from build123d import *

# Parameters (mm, degrees)
F0_W     = 350
F0_H     = 1250
F0_W_2   = 60
F0_H_2   = 48
F0_W_3   = 60.0317394733
F0_W_4   = 27
F0_H_3   = 72
F1_DEPTH = 60


with BuildPart() as f1:
    # F0 (on Front) → F1 (new body)
    with BuildSketch(Plane.XZ):
        with Locations((-0.2704625484, 126.1477753774)):
            Rectangle(F0_W, F0_H)
        with Locations((-95, -116)):
            Rectangle(F0_W_2, F0_H_2, mode=Mode.SUBTRACT)
        with Locations((-95, -49)):
            Rectangle(F0_W_2, F0_H_2, mode=Mode.SUBTRACT)
        with Locations((-95.0158697367, 18)):
            Rectangle(F0_W_3, F0_H_2, mode=Mode.SUBTRACT)
        with Locations((95, -116)):
            Rectangle(F0_W_2, F0_H_2, mode=Mode.SUBTRACT)
        with Locations((95, -49)):
            Rectangle(F0_W_2, F0_H_2, mode=Mode.SUBTRACT)
        with Locations((95.0158697367, 18)):
            Rectangle(F0_W_3, F0_H_2, mode=Mode.SUBTRACT)
        with Locations((-95.0158697367, 85)):
            Rectangle(F0_W_3, F0_H_2, mode=Mode.SUBTRACT)
        with Locations((-95.0158697367, 152)):
            Rectangle(F0_W_3, F0_H_2, mode=Mode.SUBTRACT)
        with Locations((-95.0158697367, 219)):
            Rectangle(F0_W_3, F0_H_2, mode=Mode.SUBTRACT)
        with Locations((-95.0158697367, 286)):
            Rectangle(F0_W_3, F0_H_2, mode=Mode.SUBTRACT)
        with Locations((-95.0158697367, 353)):
            Rectangle(F0_W_3, F0_H_2, mode=Mode.SUBTRACT)
        with Locations((-95, 420)):
            Rectangle(F0_W_2, F0_H_2, mode=Mode.SUBTRACT)
        with Locations((-95, 487)):
            Rectangle(F0_W_2, F0_H_2, mode=Mode.SUBTRACT)
        with Locations((-95, 554)):
            Rectangle(F0_W_2, F0_H_2, mode=Mode.SUBTRACT)
        Polygon((-0.2704625484, 669.4326684133), (12.5, 669.4326684133), (24.7295374516, 669.4326684133), (24.7295374516, 658.1978485242), (12.5, 658.1978485242), (-0.2704625484, 658.1978485242), (-25.2704625484, 658.1978485242), (-25.2704625484, 669.4326684133), align=None, mode=Mode.SUBTRACT)
        Polygon((-24.7295374516, -193.3112977796), (-24.7295374516, 639.1477753774), (25, 639.1477753774), (25, -210.8522246226), (25, -273.8522246226), (60, -273.8522246226), (60, -328.8522246226), (25, -328.8522246226), (0, -328.8522246226), (-25, -328.8522246226), (-60, -328.8522246226), (-60, -273.8522246226), (-24.7295374516, -273.8522246226), align=None, mode=Mode.SUBTRACT)
        with Locations((95.0158697367, 85)):
            Rectangle(F0_W_3, F0_H_2, mode=Mode.SUBTRACT)
        with Locations((95.0158697367, 152)):
            Rectangle(F0_W_3, F0_H_2, mode=Mode.SUBTRACT)
        with Locations((95.0158697367, 219)):
            Rectangle(F0_W_3, F0_H_2, mode=Mode.SUBTRACT)
        with Locations((95.0158697367, 286)):
            Rectangle(F0_W_3, F0_H_2, mode=Mode.SUBTRACT)
        with Locations((95.0158697367, 353)):
            Rectangle(F0_W_3, F0_H_2, mode=Mode.SUBTRACT)
        with Locations((95, 420)):
            Rectangle(F0_W_2, F0_H_2, mode=Mode.SUBTRACT)
        with Locations((95, 487)):
            Rectangle(F0_W_2, F0_H_2, mode=Mode.SUBTRACT)
        with Locations((95, 554)):
            Rectangle(F0_W_2, F0_H_2, mode=Mode.SUBTRACT)
        Polygon((174.7295374516, -540.8522246226), (174.7295374516, -498.8522246226), (-175.2704625484, -498.8522246226), (-175.2704625484, -540.8522246226), (-175.2704625484, -612.8522246226), (-175.2704625484, -648.8522246226), (174.7295374516, -648.8522246226), (174.7295374516, -612.8522246226), align=None)
        with Locations((188.2295374516, -576.8522246226)):
            Rectangle(F0_W_4, F0_H_3)
        with Locations((-188.7704625484, -576.8522246226)):
            Rectangle(F0_W_4, F0_H_3)
        Polygon((24.7295374516, 669.4326684133), (12.5, 669.4326684133), (-0.2704625484, 669.4326684133), (-25.2704625484, 669.4326684133), (-25.2704625484, 658.1978485242), (-0.2704625484, 658.1978485242), (12.5, 658.1978485242), (24.7295374516, 658.1978485242), align=None)
    extrude(amount=F1_DEPTH)


solid = f1.part
For this review, take the finished solid that the model builds, in its own axes (mm). Coordinates: 2 decimals unless noted, no trailing zeros. Order: outer loops, then holes, each group sorted by start corner. A loop starts at its lowest first (then second) coordinate and runs counter-clockwise, first axis right, second up. Notation, with made-up numbers: (74.25, 16) - (93.25, 16) arc R16 ccw to (93.25, 22) - close; hole circle Ø9 at (24.25, 38). An arc over 180 degrees is marked (long way). Use one line per item in the form item = value.
Q1. Draft analysis for pull direction Z (two halves, no side actions). For faces 1 (the flat face through (42, -60, 61)), 2 (the flat face through (-95, -30, 262)), state which applies: +Z half, -Z half, draft (parallel to the pull), parting line (faces both ways), or undercut.
Checked values:
face_1 = draft
face_2 = undercut
Q2. Consider section C-C (y = -9). Give the number of separate pieces and of enclosed holes in the cut face, then the cut area to 3 significant figures.
Checked values:
separate_pieces = 1
enclosed_holes = 23
area = 379,000 mm2
Q3. For probe 1 along X at (y, z) = (-48, -137); probe 2 along Z at (x, y) = (25.5, -46); probe 3 along X at (y, z) = (-32.5, 249), list the stretches that pass through material, from the lowest coordinate up. Write a range as from..to.
Checked values:
probe_1 = -175.27..-125, -65..-24.73, 25..65, 125..174.73
probe_2 = -648.85..-328.85, -273.85..751.15
probe_3 = -175.27..-24.73, 25..174.73
Q4. Consider section B-B (x = -40). Give the boundary of the cut face in (y, z), then the cut area to 3 significant figures.
Checked values:
outline = (-60, -648.85) - (0, -648.85) - (0, -328.85) - (-60, -328.85) - close; (-60, -273.85) - (0, -273.85) - (0, 751.15) - (-60, 751.15) - close
area = 80,700 mm2
Q5. Consider section A-A (z = -111). Give the boundary of the cut face in (x, y).
Checked values:
outline = (-175.27, -60) - (-125, -60) - (-125, 0) - (-175.27, 0) - close; (-65, -60) - (-24.73, -60) - (-24.73, 0) - (-65, 0) - close; (25, -60) - (65, -60) - (65, 0) - (25, 0) - close; (125, -60) - (174.73, -60) - (174.73, 0) - (125, 0) - close
Q6. For P1, Ø1.5, axis at y = -45, z = -31.5, coming from the +X side; P2, Ø24, axis at y = -16.5, z = 221.5, coming from the -X side; P3, Ø13.5, axis at x = 194, y = -27, coming from the +Z side, all flat-tipped, find the tip position at first contact; note any pin that passes through.
Checked values:
P1 = 174.73
P2 = -175.27
P3 = -540.85
Q7. Consider section D-D (z = -428.5). Give the boundary of the cut face in (x, y).
Checked values:
outline = (-175.27, -60) - (174.73, -60) - (174.73, 0) - (-175.27, 0) - close
